Verification items for the finished model (mm, model axes). A direction names the side the tool comes from. Round coordinates to 2 decimals unless told otherwise and drop trailing zeros. Write each loop counter-clockwise with the first axis right and the second up, starting at its lowest first coordinate (ties: lowest second). Pieces come first, ordered by that corner, then holes. Notation, with made-up numbers: (71.5, 48.5) - (124.5, 48.5) arc R13 ccw to (124.5, 67.5) - close; hole circle Ø5 at (61.5, 65). An arc over 180 degrees is marked (long way). Write each question's results on one line, items separated by ' | '.
```python
from build123d import *

# Parameters (mm, degrees)
SKETCH1_W           = 33
SKETCH1_H           = 28
BOSS_EXTRUDE1_DEPTH = 46
CUT_EXTRUDE2_DEPTH  = 59.318093247
CUT_EXTRUDE3_START  = -3
CUT_EXTRUDE3_DEPTH  = 27
FILLET1_R           = 12.5
FILLET2_R           = 16.5
FILLET3_R           = 6
SKETCH4_W           = 13
SKETCH4_H           = 23
CUT_EXTRUDE4_DEPTH  = 9
SKETCH5_R           = 6.5
CUT_EXTRUDE5_DEPTH  = 56.592265809
SKETCH6_R           = 1
CUT_EXTRUDE6_DEPTH  = 8
SKETCH7_R           = 1
SKETCH7_R_2         = 2.5
CUT_EXTRUDE7_DEPTH  = 2.5


with BuildPart() as part:
    # Sketch1 → Boss-Extrude1 (new body)
    with BuildSketch(Plane.XY):
        Rectangle(SKETCH1_W, SKETCH1_H)
    extrude(amount=BOSS_EXTRUDE1_DEPTH)

    # Sketch2 → Cut-Extrude2 (cut, through all)
    with BuildSketch(Plane(origin=(16.5, 0, 0), x_dir=(0, 0, -1), z_dir=(1, 0, 0))):
        with BuildLine():
            Line((-46, 2), (-46, -14))
            Line((-46, -14), (-5, -14))
            add(Edge.make_bspline(
                [(-5, -14), (-24.787424695, -3.854626285), (-46, 2)],
                knots=[0, 0, 0, 1, 1, 1], degree=2))
        make_face()
    extrude(amount=-CUT_EXTRUDE2_DEPTH, mode=Mode.SUBTRACT)

    # Sketch3 → Cut-Extrude3 (cut)
    with BuildSketch(Plane(origin=(16.5, 0, 0), x_dir=(0, 0, -1), z_dir=(1, 0, 0)).offset(CUT_EXTRUDE3_START)):
        with BuildLine():
            Line((-5, -14), (-2.5, -14))
            Line((-2.5, -14), (-2.5, 3.5))
            Line((-2.5, 3.5), (-40.5, 3.5))
            Line((-40.5, 3.5), (-40.5, 0.402594989))
            add(Edge.make_bspline(
                [(-5, -14), (-22.210911626, -5.175651551), (-40.5, 0.402594989)],
                knots=[0, 0, 0, 1, 1, 1], degree=2))
        make_face()
    extrude(amount=-CUT_EXTRUDE3_DEPTH, mode=Mode.SUBTRACT)

    # Fillet1
    fillet1_edges = [part.edges().sort_by_distance(p)[0] for p in [
        (13.5, 1.951297494, 40.5),
        (-13.5, 1.951297494, 40.5),
    ]]
    fillet(fillet1_edges, radius=FILLET1_R)

    # Fillet2
    fillet2_edges = [part.edges().sort_by_distance(p)[0] for p in [
        (16.5, 8, 46),
        (-16.5, 8, 46),
    ]]
    fillet(fillet2_edges, radius=FILLET2_R - 0.0001)  # a hair under: the kernel refuses the full size

    # Fillet3
    fillet3_edges = [part.edges().sort_by_distance(p)[0] for p in [
        (16.5, -14, 2.5),
        (-16.5, -14, 2.5),
    ]]
    fillet(fillet3_edges, radius=FILLET3_R)

    # Sketch4 → Cut-Extrude4 (cut)
    with BuildSketch(Plane.XZ.offset(-3.5)):
        with Locations((0, 20.5)):
            Rectangle(SKETCH4_W, SKETCH4_H)
    extrude(amount=-CUT_EXTRUDE4_DEPTH, mode=Mode.SUBTRACT)

    # Sketch5 → Cut-Extrude5 (cut, through all)
    with BuildSketch(Plane.XZ.offset(-12.5)):
        with Locations((0, 25.5)):
            Circle(SKETCH5_R)
    extrude(amount=-CUT_EXTRUDE5_DEPTH, mode=Mode.SUBTRACT)

    # Sketch6 → Cut-Extrude6 (cut)
    with BuildSketch(Plane.XZ.offset(-3.5)):
        with Locations((0, 34.3)):
            Circle(SKETCH6_R)
        with Locations((0, 6.7)):
            Circle(SKETCH6_R)
    extrude(amount=-CUT_EXTRUDE6_DEPTH, mode=Mode.SUBTRACT)

    # Sketch7 → Cut-Extrude7 (cut)
    with BuildSketch(Plane(origin=(0, 0, 0), x_dir=(-1, 0, 0), z_dir=(0, 0, -1))):
        with Locations((-9.5, 0)):
            Circle(SKETCH7_R)
        with Locations((-5, 0)):
            Circle(SKETCH7_R_2)
        with Locations((-0.5, 0)):
            Circle(SKETCH7_R)
    extrude(amount=-CUT_EXTRUDE7_DEPTH, mode=Mode.SUBTRACT)


solid = part.part
```
(1) Go/stop test with flat-tipped pins: pin 1 Ø4.5 at (x, y) = (-3, 9.5) entering from +Z; pin 2 Ø2.5 at (x, y) = (9.5, 0) entering from +Z; pin 3 Ø1.6 at (x, z) = (0, 34) entering from -Y. Record where each tip stops, or that it passes through.
Answer:
pin 1: z = 45.98 | pin 2: z = 43.21 | pin 3: y = 3.5
(2) Mould release check, pull along X, two halves, no side actions. Record for faces 4 (the cylindrical face through (-15.965, -10.476, 5.037)), 5 (the flat face through (0, -14, 1)), 6 (the flat face through (0, 11.5, 34)): released by +X, released by -X, zero draft, split by the parting line, or undercut.
Answer:
face 4: released by -X | face 5: zero draft | face 6: undercut
(3) Thickness scan on L1, parallel to Z at x = 0, y = 7.5; L2, parallel to X at y = 0.25, z = 27; L3, parallel to Y at x = 9.5, z = 2. Record the ranges inside material, lowest first.
Answer:
L1: 0 to 5.7, 7.7 to 9, 32 to 33.3, 35.3 to 46 | L2: -16.5 to -13.5, 13.5 to 16.5 | L3: -14 to -1, 1 to 14
(4) Section check A-A (z = 4). Record the cut outline in (x, y), plus the area to 3 significant figures.
Answer:
outline: (-16.5, -8) arc R6 ccw to (-13.5, -13.2) - (-13.5, 3.5) - (13.5, 3.5) - (13.5, -13.2) arc R6 ccw to (16.5, -8) - (16.5, 14) - (-16.5, 14) - close | area: 438 mm2
(5) Set-up check for faces 1 (the flat face through (5, 12.5, 31)), 2 (the cylindrical face through (2.615, 0.751, 1.232)), 3 (the cylindrical face through (15.91, -10.595, 5.037)): record each of +Z, -Z, +X, -X, +Y, -Y from which the full face is reachable in a straight line by a thin tool's end or side.
Answer:
face 1: -Y | face 2: -Z | face 3: +Z, -Z, +X, -Y
(6) Section check B-B (y = 4.75). State how many separate pieces and enclosed holes the cut face has, plus the area to 3 significant figures.
Answer:
separate pieces: 1 | enclosed holes: 3 | area: 1,100 mm2
